Could you check a few things on this model? Use its own coordinates, in mm. Face numbers are marked on the shaded views. A direction names the side the tool comes from. Give positions to 0.01 mm unless a question says otherwise; leave off trailing zeros. Order: outer loops, then holes, each group sorted by start corner. A loop starts at its lowest first (then second) coordinate and runs counter-clockwise, first axis right, second up. Notation, with made-up numbers: (87.5, -8.5) -> (111.5, -8.5) arc R6 cw to (111.5, -4.5) -> close; hole circle Ø11 at (27, 73). An arc over 180 degrees is marked (long way). Use one line per item in the form item = value. Start each with the question number.
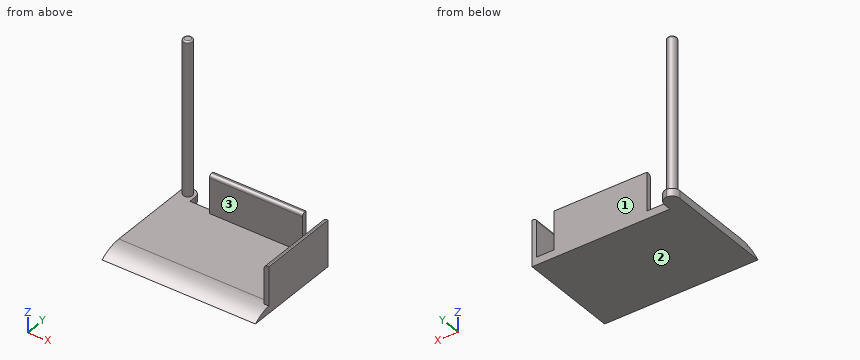
from build123d import *

# Parameters (mm, degrees)
SKETCH1_W           = 100
SKETCH1_H           = 65
BOSS_EXTRUDE2_DEPTH = 5
BOSS_EXTRUDE3_DEPTH = 10
BOSS_EXTRUDE4_DEPTH = 25
BOSS_EXTRUDE5_DEPTH = 100
FILLET1_R           = 5
FILLET2_R           = 25
FILLET5_R           = 1
SKETCH7_W           = 11.396244365786963
SKETCH7_H           = 3.3746398880239497
CUT_EXTRUDE2_DEPTH  = 25
FILLET7_R           = 2


# Some blends are built 0.0001 mm under size
with BuildPart() as part:
    # Sketch1 → Boss-Extrude2 (new body)
    with BuildSketch(Plane.XY):
        Rectangle(SKETCH1_W, SKETCH1_H)
    extrude(amount=BOSS_EXTRUDE2_DEPTH)

    # Sketch3 → Boss-Extrude3 (add)
    with BuildSketch(Plane(origin=(0, 32.499999999999986, 0), x_dir=(1, 0, 0), z_dir=(0, 1, 0))):
        Polygon((-50.00000000000001, -5), (-40.00000000000001, -5), (-40, 0), (-50.00000000000001, 0), align=None)
    extrude(amount=BOSS_EXTRUDE3_DEPTH)

    # Sketch4 → Boss-Extrude4 (add)
    with BuildSketch(Plane.XY.offset(5)):
        Polygon((49.99999999999999, 32.499999999999986), (50, -20.50000000000001), (47, -20.500000000000014), (46.99999999999999, 29.49999999999999), (-25, 29.49999999999999), (-25, 32.499999999999986), align=None)
    extrude(amount=BOSS_EXTRUDE4_DEPTH)

    # Sketch5 → Boss-Extrude5 (add)
    with BuildSketch(Plane.XY.offset(5)):
        with BuildLine():
            ThreePointArc((-48.000000000000014, 37.49999999999999), (-45.000000000000014, 34.49999999999999), (-42.000000000000014, 37.49999999999999))
            Line((-42.000000000000014, 37.49999999999999), (-45.000000000000014, 37.49999999999999))
            Line((-45.000000000000014, 37.49999999999999), (-48.000000000000014, 37.49999999999999))
        make_face()
        with BuildLine():
            Line((-45.000000000000014, 37.49999999999999), (-42.000000000000014, 37.49999999999999))
            ThreePointArc((-42.000000000000014, 37.49999999999999), (-42.87867965644041, 39.621320343559674), (-45.00000000000013, 40.49999999999999))
            Line((-45.000000000000014, 40.49999999999999), (-45.000000000000014, 37.49999999999999))
        make_face()
        with BuildLine():
            Line((-48.000000000000014, 37.49999999999999), (-45.000000000000014, 37.49999999999999))
            Line((-45.000000000000014, 37.49999999999999), (-45.000000000000014, 40.49999999999999))
            ThreePointArc((-45.00000000000013, 40.49999999999999), (-47.121320343559695, 39.621320343559596), (-48.000000000000014, 37.49999999999999))
        make_face()
    extrude(amount=BOSS_EXTRUDE5_DEPTH)

    # Fillet1
    fillet1_edges = [part.edges().sort_by_distance(p)[0] for p in [
        (-50.00000000000001, 42.499999999999986, 2.5),
        (-40, 42.499999999999986, 2.5),
    ]]
    fillet(fillet1_edges, radius=FILLET1_R - 0.0001)  # a hair under: the kernel refuses the full size

    # Fillet2
    # the kernel refuses this fillet: 25 mm, written as the material it takes off along each edge
    with BuildSketch(Plane(origin=(-87.50000000000392, -32.500000000000014, 5), x_dir=(0, 1.1369e-13, -1), z_dir=(1, 0, 0))) as fillet2_piece_1_section:
        with BuildLine():
            CenterArc((25.000000000001705, 14.999999999998728), FILLET2_R, 179.9999999999935, 36.86989764584689)
            Line((1.7053e-12, 15.00000000000157), (0, 0))
            Line((0, 0), (5.000000000000753, 0))
        make_face()
    fillet2_piece_1 = extrude(amount=175.00000000000784, mode=Mode.PRIVATE)
    fillet2_piece_1 = split(fillet2_piece_1, bisect_by=Plane(origin=(47, -26.83563604767285, 3.245395234010585), z_dir=(-1, -1.4e-16, 0)), keep=Keep.TOP, mode=Mode.PRIVATE)
    add(fillet2_piece_1, mode=Mode.SUBTRACT)
    with BuildSketch(Plane(origin=(-87.50000000000392, -32.500000000000014, 5), x_dir=(0, 1.1369e-13, -1), z_dir=(1, 0, 0))) as fillet2_piece_2_section:
        with BuildLine():
            CenterArc((25.000000000001705, 14.999999999998728), FILLET2_R, 179.9999999999935, 36.86989764584689)
            Line((1.7053e-12, 15.00000000000157), (0, 0))
            Line((0, 0), (5.000000000000753, 0))
        make_face()
    fillet2_piece_2 = extrude(amount=175.00000000000784, mode=Mode.PRIVATE)
    fillet2_piece_2 = split(fillet2_piece_2, bisect_by=Plane(origin=(48.49999999999999, -20.500000000000014, 3.245395234010585), z_dir=(1.18e-15, -1, 0)), keep=Keep.TOP, mode=Mode.PRIVATE)
    add(fillet2_piece_2, mode=Mode.SUBTRACT)

    # Fillet5
    fillet5_edges = [part.edges().sort_by_distance(p)[0] for p in [
        (-48.000000000000014, 37.49999999999999, 105),
    ]]
    fillet(fillet5_edges, radius=FILLET5_R)

    # Sketch7 → Cut-Extrude2 (cut)
    with BuildSketch(Plane.XY.offset(30.000000000000004)):
        with Locations((41.301877817106515, 31.187319944011968)):
            Rectangle(SKETCH7_W, SKETCH7_H)
    extrude(amount=-CUT_EXTRUDE2_DEPTH, mode=Mode.SUBTRACT)

    # Fillet7
    fillet7_edges = [part.edges().sort_by_distance(p)[0] for p in [
        (47, 5.999999999999986, 30),
        (5.301877817106508, 29.49999999999999, 30),
    ]]
    fillet(fillet7_edges, radius=FILLET7_R)


solid = part.part
(1) Which directions (+Z, -Z, +X, -X, +Y, -Y) give clear straight access to the entire face, cutting with the end or side of a thin tool? Please do the marked faces 1, 2 and 3.
(2) Imagine slicing it at C-C (z = 33). Write out the boundary of the cut face in (x, y).
(3) Imagine slicing it at D-D (x = 42.5). Write out the boundary of the cut face in (y, z).
(4) I'm going to push flat-ended pins straight in: pin 1 Ø8 at (x, z) = (5.5, 11) entering from +Y; pin 2 Ø1.1 at (x, y) = (49.5, -3.5) entering from +Z; pin 3 Ø3.5 at (x, z) = (49, 11.5) entering from -Y. Where does each tip first touch, or does it pass through?
(5) Imagine slicing it at B-B (y = 25). Write out the boundary of the cut face in (x, z).
(6) Imagine slicing it at A-A (x = -4.5). Write out the boundary of the cut face in (y, z), plus the area to 3 significant figures.
(7) Please list where these lines run through material, in increasing order: probe 1 along Z at (x, y) = (5.5, -2); probe 2 along Y at (x, z) = (-15, 20.5); probe 3 along X at (y, z) = (27.5, 6.5).
Calculated:
q1.face_1 = +Z, -Z, +X, +Y
q1.face_2 = -Z, +X, -X, +Y, -Y
q1.face_3 = +Z, -X, -Y
q2.outline = circle Ø6 at (-45, 37.5)
q3.outline = (-32.5, 0) -> (32.5, 0) -> (32.5, 5) -> (-17.5, 5) arc R25 ccw to start
q4.pin_1 = 32.5
q4.pin_2 = 30
q4.pin_3 = -20.5
q5.outline = (-50, 0) -> (50, 0) -> (50, 30) -> (49, 30) arc R2 ccw to (47, 28) -> (47, 5) -> (-50, 5) -> close
q6.outline = (-32.5, 0) -> (32.5, 0) -> (32.5, 30) -> (31.5, 30) arc R2 ccw to (29.5, 28) -> (29.5, 5) -> (-17.5, 5) arc R25 ccw to start
q6.area = 375 mm2
q7.probe_1 = 0 to 5
q7.probe_2 = 29.5 to 32.5
q7.probe_3 = 47 to 50
